Read the model definition and answer for the solid it produces. Units are mm, in the model's axes. A direction names the side the tool comes from. Give positions to 0.01 mm unless a question says otherwise; leave off trailing zeros. Order: outer loops, then holes, each group sorted by start corner. A loop starts at its lowest first (then second) coordinate and runs counter-clockwise, first axis right, second up.
Autodesk Fusion 360 part; units mm, degrees
sketch "Base_Sketch" plane through (0, 0, 0) normal (0, 0, 1) x (1, 0, 0)
  line L0 (-40, 44) -> (16.0721, 44)
  line L1 (16.0721, -44) -> (-40, -44)
  line L2 (-24, 5) -> (-24, 18.9991)
  line L3 (-24, -5) -> (-24, -18.9991)
  arc A0 (-27, 21.2952) -> (-24, 18.9991) centre (-24.0835, 21.9979) ccw
  line L4 (-27, 44) -> (-27, 21.2952)
  line L5 (-27, -21.2952) -> (-27, -44)
  arc A1 (-27, -17.4935) -> (-27, -17.4935) centre (-24.0728, -22.0228) ccw
  line L6 (-20, 0) -> (-20, 5)
  line L7 (-20, 5) -> (-20, 0)
  line L8 (-20, 0) -> (-20, -5)
  line L9 (-20, 5) -> (-24, 5)
  line L10 (-20, -5) -> (-24, -5)
  circle A2 centre (-46, 0.0012) radius 9.5
  arc A3 (-45.4349, 18.9928) -> (-45.4349, -18.9904) centre (-46, 0.0012) ccw
  arc A4 (-45.4349, 18.9928) -> (-40, 23.5243) centre (-45.8206, 24.9804) ccw
  line L11 (-40, -44) -> (-40, -23.5218)
  line L12 (-40, 23.5243) -> (-40, 44)
  arc A5 (-40, -23.5218) -> (-45.4349, -18.9904) centre (-45.8206, -24.978) ccw
  arc A6 (-24, -18.9991) -> (-27, -21.2952) centre (-24.0835, -21.9979) ccw
  arc A7 (50.0608, -16.1177) -> (50.0608, 16.1177) centre (40, 0) ccw
  circle A8 centre (4, 25) radius 5
  circle A9 centre (4, -25) radius 5
  line L13 (50.0608, -16.1177) -> (21.0769, -42.0859)
  arc A10 (16.0721, -44) -> (21.0769, -42.0859) centre (16.0721, -36.5) ccw
  line L14 (50.0608, 16.1177) -> (21.0769, 42.0859)
  arc A11 (21.0769, 42.0859) -> (16.0721, 44) centre (16.0721, 36.5) ccw
  dimension "d3" = 13
  dimension "d7" = 3
  dimension "d9" = 4
  dimension "d11" = 19
  dimension "d12" = 38
  dimension "d13" = 12
  dimension "d14" = 38
  dimension "d19" = 10
  dimension "d22" = 7.5
extrude "Extrude1" add sketch "Base_Sketch" along normal blind 10 contours L0 L1 L2 L3 A0 L4 L5 A1 L6 L7 L8 L9 L10 A7 L13 A10 L14 A11 | L3 L5 A1 A6 picked at (-23.8485, -22.1321)
extrude "Extrude2" add sketch "Base_Sketch" along normal blind 50 contours L0 L1 L2 L3 A0 L4 L5 A1 L6 L7 L8 L9 L10 A3 A4 L11 L12 A5 | L3 L5 A1 A6 picked at (-28.5466, -20.9909)
sketch "Triangle_Sketch" plane through (0, 0, 0) normal (0, 1, 0) x (1, 0, 0)
  line L0 (-20, -50) -> (-20, -10)
  line L1 (-20, -10) -> (40, -10)
  line L2 (40, -10) -> (-20, -50)
  dimension "d27" = 60
extrude "Extrude3" add sketch "Triangle_Sketch" along normal mid plane 10
1) Consider L1, parallel to Y at x = 4, z = 7; L2, parallel to Y at x = -46, z = 16.5; L3, parallel to Y at x = 16.5, z = 18.5. Determine where each line is inside the solid, lowest interval first.
Final values:
L1: y = -44 to -30, -20 to 20, 30 to 44
L2: y = -19 to -9.5, 9.5 to 19
L3: y = -5 to 5
2) For a pull along Y with two mould halves and no side action, classify faces 1 (the face through (59, 0, 5)), 2 (the face through (-42.019, -20.336, 24.65)), 3 (the face through (-37.224, 3.64, 24.65)) as released by +Y, released by -Y, zero draft, split by the parting line, or undercut.
Final values:
face 1: split by the parting line
face 2: released by -Y
face 3: undercut
3) Given pin 1 (2 mm diameter, centred on y = 34, z = 10, fed in from -X); pin 2 (9 mm diameter, centred on x = 4, y = 25, fed in from +Z); pin 3 (1.5 mm diameter, centred on x = 4, z = 19, fed in from +Y); pin 4 (15.5 mm diameter, centred on y = -14.5, z = 30, fed in from +X), each flat-ended and moving along its own axis, determine where each tip first touches the part or whether it passes through.
Final values:
pin 1: stops at x = -40
pin 2: passes through
pin 3: stops at y = 5
pin 4: stops at x = -24
4) The part is cut by section B-B on z = 5.5. Determine the outline of the cut face in (x, y).
Final values:
outline: (-45.43, -18.99) arc R6 cw to (-40, -23.52) - (-40, -44) - (16.07, -44) arc R7.5 ccw to (21.08, -42.09) - (50.06, -16.12) arc R19 ccw to (50.06, 16.12) - (21.08, 42.09) arc R7.5 ccw to (16.07, 44) - (-40, 44) - (-40, 23.52) arc R6 cw to (-45.43, 18.99) arc R19 ccw (long way) to start; hole circle Ø19 at (-46, 0); hole circle Ø10 at (4, -25); hole circle Ø10 at (4, 25)
5) The part is cut by section D-D on z = 41. Determine the outline of the cut face in (x, y), and give its area (3 significant figures).
Final values:
outline: (-45.43, -18.99) arc R6 cw to (-40, -23.52) - (-40, -44) - (-27, -44) - (-27, -21.3) arc R3 cw to (-24, -19) - (-24, -5) - (-6.5, -5) - (-6.5, 5) - (-24, 5) - (-24, 19) arc R3 cw to (-27, 21.3) - (-27, 44) - (-40, 44) - (-40, 23.52) arc R6 cw to (-45.43, 18.99) arc R19 ccw (long way) to start; hole circle Ø19 at (-46, 0)
area: 1,960 mm2
6) The part is cut by section A-A on x = 4. Determine the outline of the cut face in (y, z).
Final values:
outline: (-44, 0) - (-30, 0) - (-30, 10) - (-44, 10) - close; (-20, 0) - (20, 0) - (20, 10) - (5, 10) - (5, 34) - (-5, 34) - (-5, 10) - (-20, 10) - close; (30, 0) - (44, 0) - (44, 10) - (30, 10) - close
7) The part is cut by section C-C on x = -51. Determine the outline of the cut face in (y, z), and give its area (3 significant figures).
Final values:
outline: (-18.33, 0) - (-8.08, 0) - (-8.08, 50) - (-18.33, 50) - close; (8.08, 0) - (18.33, 0) - (18.33, 50) - (8.08, 50) - close
area: 1,030 mm2
8) A tool of negligible diameter and unlimited length cuts with its end or side. For faces 4 (the face through (-24, -12, 30)), 5 (the face through (-40, 34, 25)), 6 (the face through (-24, 12, 30)), 7 (the face through (-40, -34, 25)), from which of +Z, -Z, +X, -X, +Y, -Y can it reach the whole face along a straight path? Write none if from no direction.
Final values:
face 4: +Z, +X, -Y
face 5: +Z, -Z, -X, +Y
face 6: +Z, +X, +Y
face 7: +Z, -Z, -X, -Y
